Part model, mm, in its own coordinate system. A direction names the side the tool comes from. Round coordinates to 2 decimals unless told otherwise and drop trailing zeros. Loops run counter-clockwise (first coordinate to the right, second up) from the corner with the lowest first, then second, coordinate; pieces in that order, holes last. Notation, with made-up numbers: (54, 51.25) - (73, 51.25) arc R22 cw to (73, 77.25) - close; hole circle Ø2 at (9, 83.5). An arc over 180 degrees is marked (long way). Write each question's results on one line, items separated by ' | '. Start each with the question number.
(1) Cut at C-C, the plane x = -0.5. List the corners of the cut face in (y, z), then the cut area to 3 significant figures.
(2) Cut at A-A, the plane z = 0. List the corners of the cut face in (x, y), then the cut area to 3 significant figures.
(3) Cut at D-D, the plane z = 3.25. List the corners of the cut face in (x, y).
(4) Cut at B-B, the plane y = 33.5. List the corners of the cut face in (x, z).
(5) Flat gauge pins, fed straight in: P1, Ø1, axis at x = 1, z = -2, coming from the -Y side; P2, Ø1, axis at x = -2.5, z = 3, coming from the +Y side. Where does each tip first touch, or does it go through?
(6) Tool access for faces 1 (the face through (-2, 40.21, 2)), 2 (the face through (-3.464, 20, 0)): list every direction of +Z, -Z, +X, -X, +Y, -Y with a clear straight run to the whole face (end or side of a thin tool).
(7) Drill centre lines: L1, parallel to Y at x = 0, z = 3.75; L2, parallel to Z at x = 1.25, y = 10; L3, parallel to X at y = 31, z = 2.5. Where is each one in solid material? Low to high.
from build123d import *

# Parameters (mm, degrees)
BOSS_EXTRUDE1_DEPTH      = 40.21
SKETCH2_R                = 2.25
BOSS_EXTRUDE2_DEPTH      = 3
BOSS_EXTRUDE2_DEPTH_BACK = 30


with BuildPart() as part:
    # Sketch1 → Boss-Extrude1 (new body)
    with BuildSketch(Plane(origin=(0, 0, 0), x_dir=(1, 0, 0), z_dir=(0, 1, 0))):
        Polygon((0, -4), (3.464101615, -2), (3.464101615, 2), (0, 4), (-3.464101615, 2), (-3.464101615, -2), align=None)
    extrude(amount=BOSS_EXTRUDE1_DEPTH)

    # Sketch2 → Boss-Extrude2 (add, two sides)
    with BuildSketch(Plane(origin=(0, 40.21, 0), x_dir=(1, 0, 0), z_dir=(0, 1, 0))) as boss_extrude2_sk:
        Circle(SKETCH2_R)
    extrude(amount=BOSS_EXTRUDE2_DEPTH)
    extrude(boss_extrude2_sk.sketch, amount=-BOSS_EXTRUDE2_DEPTH_BACK)


solid = part.part
A:
1) outline: (0, -3.71) - (40.21, -3.71) - (40.21, -2.19) - (43.21, -2.19) - (43.21, 2.19) - (40.21, 2.19) - (40.21, 3.71) - (0, 3.71) - close | area: 312 mm2
2) outline: (-3.46, 0) - (3.46, 0) - (3.46, 40.21) - (2.25, 40.21) - (2.25, 43.21) - (-2.25, 43.21) - (-2.25, 40.21) - (-3.46, 40.21) - close | area: 292 mm2
3) outline: (-1.3, 0) - (1.3, 0) - (1.3, 40.21) - (-1.3, 40.21) - close
4) outline: (-3.46, -2) - (0, -4) - (3.46, -2) - (3.46, 2) - (0, 4) - (-3.46, 2) - close
5) P1: y = 0 | P2: y = 40.21
6) face 1: +Y | face 2: +Z, -Z, -X, +Y, -Y
7) L1: 0 to 40.21 | L2: -3.28 to 3.28 | L3: -2.6 to 2.6
